Could you check a few things on this model? Use its own coordinates, in mm. A direction names the side the tool comes from. Round coordinates to 2 decimals unless told otherwise and drop trailing zeros. Loops run counter-clockwise (first coordinate to the right, second up) from the corner with the lowest first, then second, coordinate; pieces in that order, holes last. Notation, with made-up numbers: (20, 45) - (65, 45) arc R15 cw to (65, 54) - close; hole circle Ø6 at (-33.75, 68.25). An arc over 180 degrees is marked (long way). Use one line per item in the form item = value.
```python
from build123d import *

# Parameters (mm, degrees)
SKETCH_1_W          = 68.2
SKETCH_1_H          = 17.95
EXTRUDE_1_DEPTH     = 3.5
SKETCH_21_W         = 68.2
SKETCH_21_H         = 3.5
EXTRUDE_4_DEPTH     = 28.25
SKETCH_24_R         = 2.85
CUT_EXTRUDE_2_DEPTH = 28.25


with BuildPart() as part:
    # 草圖1 → 1 (new body)
    with BuildSketch(Plane.XY):
        Rectangle(SKETCH_1_W, SKETCH_1_H)
    extrude(amount=EXTRUDE_1_DEPTH)

    # 草圖21 → 填料-伸長4 (add)
    with BuildSketch(Plane.XY.offset(3.5)):
        with Locations((0, 7.225)):
            Rectangle(SKETCH_21_W, SKETCH_21_H)
    extrude(amount=EXTRUDE_4_DEPTH)

    # 草圖24 → 除料-伸長2 (cut)
    with BuildSketch(Plane(origin=(0, 0, 0), x_dir=(-1, 0, 0), z_dir=(0, 0, -1))):
        with Locations((0, -3.070533486)):
            Circle(SKETCH_24_R)
    extrude(amount=-CUT_EXTRUDE_2_DEPTH, mode=Mode.SUBTRACT)


solid = part.part
```
1. If we section it at D-D, the plane z = 28: Write out the boundary of the cut face in (x, y) (3 decimals).
Solution:
outline = (-34.1, 5.475) - (34.1, 5.475) - (34.1, 8.975) - (-34.1, 8.975) - close
2. If we section it at A-A, the plane x = 0: Write out the boundary of the cut face in (y, z) (3 decimals), plus the area to 3 significant figures.
Solution:
outline = (-8.975, 0) - (-5.921, 0) - (-5.921, 3.5) - (-8.975, 3.5) - close; (-0.221, 0) - (8.975, 0) - (8.975, 31.75) - (5.475, 31.75) - (5.475, 3.5) - (-0.221, 3.5) - close
area = 142 mm^2
3. On a 3-axis mill with a long thin cutter (end or side, diameter ignored), from which of +Z, -Z, +X, -X, +Y, -Y can I reach the whole of each face in a straight line? I mean faces 1 (the face through (0, 0, 0)), 2 (the face through (0, 5.475, 17)). Say none if no direction works.
Solution:
face_1 = -Z, +X, -X, +Y, -Y
face_2 = +Z, +X, -X, -Y
4. We'd pull the mould along X, two halves only. Please class faces 3 (the face through (34.1, 6, 11)), 4 (the face through (0, 7, 31.75)), 5 (the face through (-34.1, 6, 11)), 6 (the face through (2.262, -4.805, 1.726)): +X half, -X half, draft (parallel to the pull), parting line (faces both ways), or undercut.
Solution:
face_3 = +X half
face_4 = draft
face_5 = -X half
face_6 = undercut
5. Please list where these lines run through material, in increasing order: line 1 along Y through (x, z) = (0, 1.3) (3 decimals); line 2 along Y through (x, z) = (10, 9) (3 decimals); line 3 along Z through (x, y) = (17.5, -5.5).
Solution:
line_1 = -8.975 to -5.921, -0.221 to 8.975
line_2 = 5.475 to 8.975
line_3 = 0 to 3.5
6. If we section it at C-C, the plane y = 3: Write out the boundary of the cut face in (x, z).
Solution:
outline = (-34.1, 0) - (34.1, 0) - (34.1, 3.5) - (-34.1, 3.5) - close
7. For P1, Ø3, axis at x = 12, z = 24.5, coming from the -Y side (3 decimals); P2, Ø5, axis at x = 0, y = -3.07, coming from the -Z side; P3, Ø3, axis at x = 18.5, y = -1.5, coming from the -Z side, each with a flat end and sliding along its axis, tell me the tip position at first contact or that it passes through.
Solution:
P1 = 5.475
P2 = through
P3 = 0
8. If we section it at B-B, the plane x = 23: Write out the boundary of the cut face in (y, z) (3 decimals).
Solution:
outline = (-8.975, 0) - (8.975, 0) - (8.975, 31.75) - (5.475, 31.75) - (5.475, 3.5) - (-8.975, 3.5) - close
